```python
from build123d import *

# Parameters (mm, degrees)
SKETCH1_R              = 5.2324
BOSS_EXTRUDE1_DEPTH    = 3.175
SKETCH2_W              = 65.151
SKETCH2_H              = 3.175
BOSS_EXTRUDE2_DEPTH    = 25.4
FILLET1_R              = 2.54
CUT_EXTRUDE1_DEPTH     = 3.175
CONVERT_SOLID1_START   = -32.6263
CONVERT_SOLID1_DEPTH   = 65.151
CONVERT_SOLID1_2_DEPTH = 65.151


# Read off the part's stored shape, not the designer's step: Convert-Solid1
with BuildPart() as part:
    # Sketch1 → Boss-Extrude1 (new body)
    with BuildSketch(Plane.XY):
        with BuildLine():
            Line((32.5247, -81.185268118), (32.5247, -14.510268118))
            ThreePointArc((32.5247, -14.510268118), (23.7617, -5.747268118), (14.9987, -14.510268118))
            ThreePointArc((14.9987, -14.510268118), (-0.0508, -29.559768118), (-15.1003, -14.510268118))
            ThreePointArc((-15.1003, -14.510268118), (-23.8633, -5.747268118), (-32.6263, -14.510268118))
            Line((-32.6263, -14.510268118), (-32.6263, -81.185268118))
            Line((-32.6263, -81.185268118), (32.5247, -81.185268118))
        make_face()
        with Locations((-23.8633, -14.510268118)):
            Circle(SKETCH1_R, mode=Mode.SUBTRACT)
        with Locations((23.7617, -14.510268118)):
            Circle(SKETCH1_R, mode=Mode.SUBTRACT)
    extrude(amount=BOSS_EXTRUDE1_DEPTH)

    # Sketch2 → Boss-Extrude2 (add)
    with BuildSketch(Plane(origin=(0, 0, 0), x_dir=(-1, 0, 0), z_dir=(0, 0, -1))):
        with Locations((0.0508, -79.597768118)):
            Rectangle(SKETCH2_W, SKETCH2_H)
    extrude(amount=BOSS_EXTRUDE2_DEPTH)

    # Fillet1
    fillet1_edges = [part.edges().sort_by_distance(p)[0] for p in [
        (32.5247, -79.597768118, -25.4),
        (-32.6263, -79.597768118, -25.4),
    ]]
    fillet(fillet1_edges, radius=FILLET1_R)

    # Sketch3 → Cut-Extrude1 (cut)
    with BuildSketch(Plane(origin=(0, -78.010268118, 0), x_dir=(1, 0, 0), z_dir=(0, 1, 0))):
        with BuildLine():
            Line((15.538165915, 12.554273752), (15.538165915, 17.634273752))
            ThreePointArc((15.538165915, 17.634273752), (19.705353415, 21.801461252), (23.872540915, 17.634273752))
            Line((23.872540915, 17.634273752), (23.872540915, 12.554273752))
            ThreePointArc((23.872540915, 12.554273752), (19.705353415, 8.387086252), (15.538165915, 12.554273752))
        make_face()
        with BuildLine():
            Line((-24.461834085, 12.554273752), (-24.461834085, 17.634273752))
            ThreePointArc((-24.461834085, 17.634273752), (-20.294646585, 21.801461252), (-16.127459085, 17.634273752))
            Line((-16.127459085, 17.634273752), (-16.127459085, 12.554273752))
            ThreePointArc((-16.127459085, 12.554273752), (-20.294646585, 8.387086252), (-24.461834085, 12.554273752))
        make_face()
    extrude(amount=-CUT_EXTRUDE1_DEPTH, mode=Mode.SUBTRACT)

    # Convert-Solid1 outline → Convert-Solid1 (cut)
    with BuildSketch(Plane.YZ.offset(CONVERT_SOLID1_START)):
        with BuildLine():
            Line((-81.185268118, 3.175), (-81.185268118, -3.175))
            ThreePointArc((-81.185268118, -3.175), (-79.325396179, 1.315128061), (-74.835268118, 3.175))
            Line((-74.835268118, 3.175), (-81.185268118, 3.175))
        make_face()
    extrude(amount=CONVERT_SOLID1_DEPTH, mode=Mode.SUBTRACT)

    # Convert-Solid1 2 outline → Convert-Solid1 2 (add)
    with BuildSketch(Plane.YZ.offset(CONVERT_SOLID1_START)):
        with BuildLine():
            Line((-78.010268118, 0), (-78.010268118, -3.175))
            ThreePointArc((-78.010268118, -3.175), (-77.080332148, -0.92993597), (-74.835268118, 0))
            Line((-74.835268118, 0), (-78.010268118, 0))
        make_face()
    extrude(amount=CONVERT_SOLID1_2_DEPTH)


solid = part.part
```
Source: CAD feature listing. Evaluate the final solid. Frame: model axes, mm. A direction names the side the tool comes from. Coordinates: 2 decimals unless noted, no trailing zeros. Loops run counter-clockwise (first coordinate to the right, second up) from the corner with the lowest first, then second, coordinate; pieces in that order, holes last. Notation, with made-up numbers: M 71,32 L 114,32 A28 cw 114,69 Z; hole C 24,29.25 d6. An arc over 180 degrees is marked long. Use a Markdown table: item, result. Add a question column.
Q1. Material intervals for L1, parallel to Z at x = -26.5, y = -63.5 (3 decimals); L2, parallel to Y at x = 5, z = -17; L3, parallel to Y at x = 21.5, z = 1, sorted ascending.
Q2. Section query A-A, the plane y = -21. Return loops of the section in (x, z) (3 decimals).
Q3. Section query B-B, the plane z = -19. Return loops of the section in (x, y).
Q4. Draft query along X for faces 4 (the flat face through (32.525, -55, 1)), 5 (the flat face through (0, -81.185, -14)), 6 (the flat face through (-32.626, -55, 1)), 7 (the flat face through (23.873, -80, -15)). Return one class per face: pulls with the +X half, pulls with the -X half, needs draft (parallel to the pull), parting line crosses it, or undercut.
Q5. First-contact query: pin 1 (19.5 mm diameter, centred on x = -7.5, y = -44.5, fed in from -Z); pin 2 (6.5 mm diameter, centred on x = -4.5, z = -11.5, fed in from +Y); pin 3 (3 mm diameter, centred on x = -15, z = -4, fed in from +Y). Flat tips, straight axial feed; report the tip coordinate or a pass-through.
Q6. Access query for faces 1 (the cylindrical face through (19.6, -79.6, -21.8)), 2 (the flat face through (0, -78.01, -14)), 3 (the cylindrical face through (23.95, -5.75, 1.57)). Directions: +Z, -Z, +X, -X, +Y, -Y. A direction counts if a zero-diameter tool reaches every point of the face in a straight line with its end or side. Return the directions, or none.
Q7. Section query D-D, the plane x = -21. Return loops of the section in (y, z) (3 decimals), and give its area (3 significant figures).
Result:
| question | item | result |
|---|---|---|
| 1 | L1 | z = 0 to 3.175 |
| 1 | L2 | y = -81.19 to -78.01 |
| 1 | L3 | y = -79.62 to -19.23, -9.79 to -6.04 |
| 2 | outline | M -32.626,0 L -13.629,0 L -13.629,3.175 L -32.626,3.175 Z; M 13.528,0 L 32.525,0 L 32.525,3.175 L 13.528,3.175 Z |
| 3 | outline | M -32.63,-81.19 L -24.23,-81.19 L -24.23,-78.01 L -32.63,-78.01 Z; M -16.36,-81.19 L 15.77,-81.19 L 15.77,-78.01 L -16.36,-78.01 Z; M 23.64,-81.19 L 32.52,-81.19 L 32.52,-78.01 L 23.64,-78.01 Z |
| 4 | face 4 | pulls with the +X half |
| 4 | face 5 | needs draft |
| 4 | face 6 | pulls with the -X half |
| 4 | face 7 | undercut |
| 5 | pin 1 | stops at z = 0 |
| 5 | pin 2 | stops at y = -78.01 |
| 5 | pin 3 | stops at y = -77.94 |
| 6 | face 1 | +Y, -Y |
| 6 | face 2 | -Z, +X, -X, +Y |
| 6 | face 3 | +Z, -Z, +Y |
| 7 | outline | M -81.185,-25.4 L -78.01,-25.4 L -78.01,-21.741 L -81.185,-21.741 Z; M -81.185,-8.447 L -78.01,-8.447 L -78.01,-3.175 A3.175 cw -74.835,0 L -18.89,0 L -18.89,3.175 L -74.835,3.175 A6.35 ccw -81.185,-3.175 Z; M -10.131,0 L -6.228,0 L -6.228,3.175 L -10.131,3.175 Z |
| 7 | area | 242 mm2 |
